from build123d import *

# Parameters (mm, degrees)
SKETCH_1_R          = 22.35
EXTRUDE_1_DEPTH     = 3.5
CUT_EXTRUDE_START   = 3.5
CUT_EXTRUDE_1_DEPTH = 3.5
CHAMFER_1_SIZE      = 0.5
CUT_EXTRUDE_2_DEPTH = 3.5
FILLET_1_R          = 0.5
CHAMFER_2_SIZE      = 0.25
CUT_EXTRUDE_3_DEPTH = 2
FILLET_2_R          = 0.3


with BuildPart() as part:
    # 草图1 → 凸台-拉伸1 (new body)
    with BuildSketch(Plane.XY):
        Circle(SKETCH_1_R)
    extrude(amount=EXTRUDE_1_DEPTH)

    # 草图2 → 切除-拉伸1 (cut)
    with BuildSketch(Plane.XY.offset(CUT_EXTRUDE_START)):
        with BuildLine():
            Line((-5.5, 0), (-5.5, 5.5))
            ThreePointArc((-5.5, 5.5), (-5.207106781, 6.207106781), (-4.5, 6.5))
            Line((-4.5, 6.5), (4.5, 6.5))
            ThreePointArc((4.5, 6.5), (5.207106781, 6.207106781), (5.5, 5.5))
            Line((5.5, 5.5), (5.5, -3.85))
            ThreePointArc((5.5, -3.85), (5.207106781, -4.557106781), (4.5, -4.85))
            Line((4.5, -4.85), (-4.5, -4.85))
            ThreePointArc((-4.5, -4.85), (-5.207106781, -4.557106781), (-5.5, -3.85))
            Line((-5.5, -3.85), (-5.5, 0))
        make_face()
    extrude(amount=-CUT_EXTRUDE_1_DEPTH, mode=Mode.SUBTRACT)

    # 倒角1
    chamfer_1_edges = [part.edges().sort_by_distance(p)[0] for p in [
        (-22.35, 0, 3.5),
    ]]
    chamfer(chamfer_1_edges, length=CHAMFER_1_SIZE)

    # 草图3 → 切除-拉伸2 (cut)
    with BuildSketch(Plane.XY.offset(CUT_EXTRUDE_START)):
        Polygon((0, 6.5), (-4.1, 6.5), (-4.1, 8.5), (4.1, 8.5), (4.1, 6.5), align=None)
    extrude(amount=-CUT_EXTRUDE_2_DEPTH, mode=Mode.SUBTRACT)

    # 圆角1
    fillet_1_edges = [part.edges().sort_by_distance(p)[0] for p in [
        (4.1, 6.5, 1.75),
        (-4.1, 6.5, 1.75),
        (4.1, 8.5, 1.75),
        (-4.1, 8.5, 1.75),
    ]]
    fillet(fillet_1_edges, radius=FILLET_1_R)

    # 倒角2
    chamfer_2_edges = [part.edges().sort_by_distance(p)[0] for p in [
        (-5.5, 0.825, 0),
        (0, -4.85, 0),
        (5.5, 0.825, 0),
        (-5.230296743, 6.183130051, 0),
        (5.207106781, -4.557106781, 0),
        (-5.207106781, -4.557106781, 0),
        (4.1, 7.498331477, 0),
        (5.230296743, 6.183130051, 0),
        (-4.1, 7.498331477, 0),
        (0, 8.5, 0),
        (-4.234851628, 6.655097929, 0),
        (4.234851628, 6.655097929, 0),
        (3.953553391, 8.353553391, 0),
        (-3.953553391, 8.353553391, 0),
    ]]
    chamfer(chamfer_2_edges, length=CHAMFER_2_SIZE)

    # 草图4 → 切除-拉伸3 (cut)
    with BuildSketch(Plane.XY.offset(CUT_EXTRUDE_START)):
        with BuildLine():
            Line((-2, 20.7), (-2, 19.7))
            Line((-2, 19.7), (-2, 14.3))
            Line((-2, 14.3), (0, 14.3))
            Line((0, 14.3), (2, 14.3))
            Line((2, 14.3), (2, 19.7))
            Line((2, 19.7), (2, 20.7))
            ThreePointArc((2, 20.7), (0, 20.801262586), (-2, 20.7))
        make_face()
    extrude(amount=-CUT_EXTRUDE_3_DEPTH, mode=Mode.SUBTRACT)

    # 圆角2
    fillet_2_edges = [part.edges().sort_by_distance(p)[0] for p in [
        (-2, 20.7, 2.5),
        (2, 20.7, 2.5),
        (2, 14.3, 2.5),
        (-2, 14.3, 2.5),
    ]]
    fillet(fillet_2_edges, radius=FILLET_2_R)


solid = part.part
Read the model definition and answer for the solid it produces. Units are mm, in the model's axes. A direction names the side the tool comes from. Coordinates: 2 decimals unless noted, no trailing zeros. Loops run counter-clockwise (first coordinate to the right, second up) from the corner with the lowest first, then second, coordinate; pieces in that order, holes last. Notation, with made-up numbers: (57, 47.25) -> (93, 47.25) arc R14 ccw to (93, 52.25) -> close; hole circle Ø3 at (7, -39). An arc over 180 degrees is marked (long way). Answer in a Markdown table with one row per item.
Item 1: A cutting plane is placed at B-B on x = 0. Determine the outline of the cut face in (y, z).
Returned:
| item | result |
|---|---|
| outline | (-22.35, 0) -> (-5.1, 0) -> (-4.85, 0.25) -> (-4.85, 3.5) -> (-21.85, 3.5) -> (-22.35, 3) -> close; (8.5, 0.25) -> (8.75, 0) -> (22.35, 0) -> (22.35, 3) -> (21.85, 3.5) -> (20.8, 3.5) -> (20.8, 1.5) -> (14.3, 1.5) -> (14.3, 3.5) -> (8.5, 3.5) -> close |
Item 2: Each of these flat-tipped pins is pushed along its axis until it touches: P1, Ø0.5, axis at y = 7.5, z = 2, coming from the -X side; P2, Ø2, axis at x = 0.5, y = 18, coming from the +Z side; P3, Ø1, axis at x = -1.5, z = 1.5, coming from the -Y side; P4, Ø1, axis at x = -16.5, y = -18, coming from the -Z side. Where does it stop, or does it pass through?
Returned:
| item | result |
|---|---|
| P1 | stops at x = -21.14 |
| P2 | stops at z = 1.5 |
| P3 | stops at y = -22.33 |
| P4 | passes through |
Item 3: For a pull along Y with two mould halves and no side action, classify faces 4 (the cylindrical face through (5.215, -4.549, 1.898)), 5 (the cylindrical face through (-2.91, 22.16, 1.48)) as released by +Y, released by -Y, zero draft, split by the parting line, or undercut.
Returned:
| item | result |
|---|---|
| face 4 | undercut |
| face 5 | split by the parting line |
Item 4: A cutting plane is placed at A-A on y = 0. Determine the outline of the cut face in (x, z).
Returned:
| item | result |
|---|---|
| outline | (-22.35, 0) -> (-5.75, 0) -> (-5.5, 0.25) -> (-5.5, 3.5) -> (-21.85, 3.5) -> (-22.35, 3) -> close; (5.5, 0.25) -> (5.75, 0) -> (22.35, 0) -> (22.35, 3) -> (21.85, 3.5) -> (5.5, 3.5) -> close |
Item 5: For faces 1 (the cylindrical face through (5.223, 6.191, 1.898)), 2 (the conical face through (5.312, 6.276, 0.127)), 3 (the flat face through (-2, 18, 3)), determine the directions among +Z, -Z, +X, -X, +Y, -Y from which every point of the face is accessible in a straight line to the end or side of a thin tool.
Returned:
| item | result |
|---|---|
| face 1 | +Z, -Z |
| face 2 | -Z |
| face 3 | +Z |
Item 6: Straight lines are drawn through the part: line 1 along Y through (x, z) = (0.5, 1.8); line 2 along X through (y, z) = (0.5, 2.8); line 3 along X through (y, z) = (16, 3.25) (3 decimals). For each, find the intervals that lie inside material, in ascending order. Write a range as [from, to].
Returned:
| item | result |
|---|---|
| line 1 | y = [-22.34, -4.85], [8.5, 14.3], [20.79, 22.34] |
| line 2 | x = [-22.34, -5.5], [5.5, 22.34] |
| line 3 | x = [-15.245, -2], [2, 15.245] |
